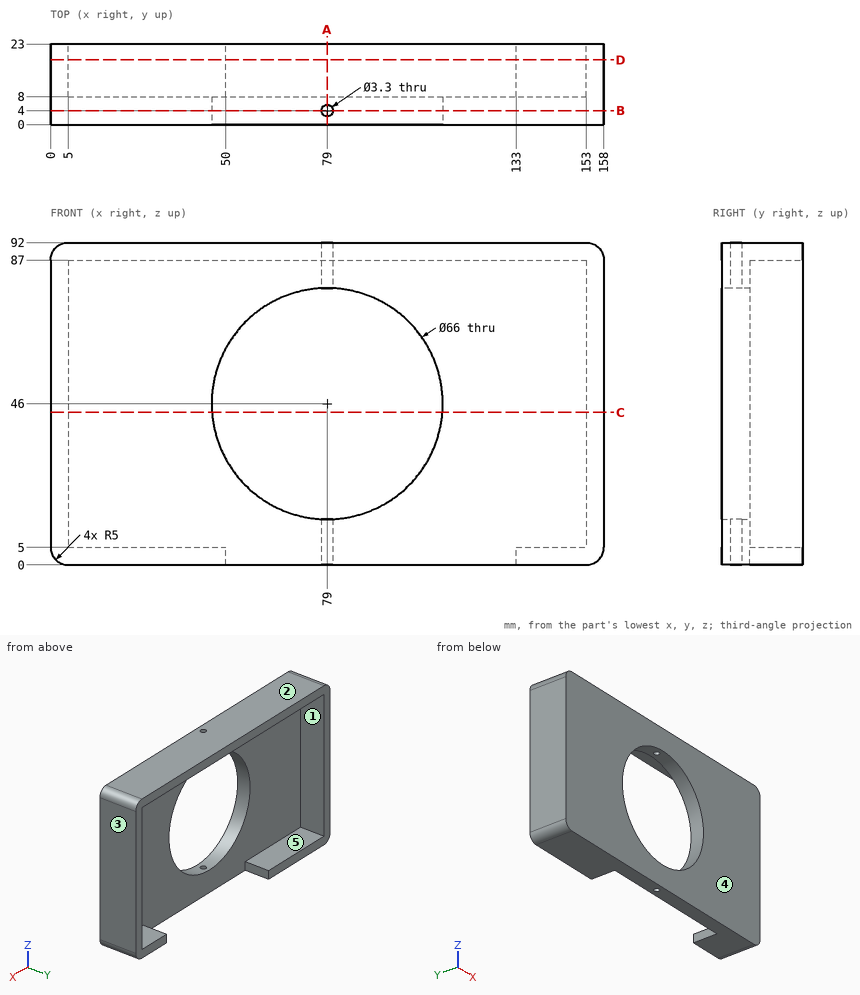
Part print with two shaded views. Sizes in mm from the minimum x, y, z corner. A direction names the side the tool comes from. Round coordinates to 2 decimals unless told otherwise and drop trailing zeros. Order: outer loops, then holes, each group sorted by start corner. A loop starts at its lowest first (then second) coordinate and runs counter-clockwise, first axis right, second up.
(1) Pull direction X, two halves, no side cores. Call the marked faces 1, 2 and 3: released by +X, released by -X, zero draft, split by the parting line, or undercut.
(2) Band-saw the part on A-A (x = 79). List the corners of the cut face in (y, z), then the cut area to 3 significant figures.
(3) 3-axis set-ups, long thin cutter, end or side, ignore diameter. For the marked faces 4 and 5: which of +Z, -Z, +X, -X, +Y, -Y reach the whole face in a straight line?
(4) Band-saw the part on B-B (y = 4). List the corners of the cut face in (x, z), then the cut area to 3 significant figures.
(5) Drill centre lines: line 1 (Y direction, x = 79, z = 10); line 2 (Z direction, x = 29, y = 17); line 3 (X direction, y = 11.5, z = 73.5). Where is each one in solid material? Low to high.
(6) Band-saw the part on C-C (z = 43.5). List the corners of the cut face in (x, y).
(7) Pin check, flat tips, straight feed: pin 1 (5.5 mm diameter, centred on y = 12.5, z = 1.5, fed in from +X); pin 2 (5.5 mm diameter, centred on y = 16, z = 1.5, fed in from -X); pin 3 (6 mm diameter, centred on x = 16, z = 20.5, fed in from +Y). Stop position of each tip, or through.
(8) Band-saw the part on D-D (y = 18.5). List the corners of the cut face in (x, z).
Verdict:
1. face 1: undercut
1. face 2: zero draft
1. face 3: released by +X
2. outline: (0, 0) - (2.35, 0) - (2.35, 13) - (0, 13) - close; (0, 79) - (2.35, 79) - (2.35, 92) - (0, 92) - close; (5.65, 0) - (8, 0) - (8, 13) - (5.65, 13) - close; (5.65, 79) - (8, 79) - (8, 87) - (23, 87) - (23, 92) - (5.65, 92) - close
2. area: 197 mm2
3. face 4: +Z, -Z, +X, -X, -Y
3. face 5: +Y
4. outline: (0, 5) arc R5 ccw to (5, 0) - (77.35, 0) - (77.35, 13.04) arc R33 cw to (77.35, 78.96) - (77.35, 92) - (5, 92) arc R5 ccw to (0, 87) - close; (80.65, 0) - (153, 0) arc R5 ccw to (158, 5) - (158, 87) arc R5 ccw to (153, 92) - (80.65, 92) - (80.65, 78.96) arc R33 cw to (80.65, 13.04) - close
4. area: 11,000 mm2
5. line 1: y = 0 to 2.35, 5.65 to 8
5. line 2: z = 0 to 5, 87 to 92
5. line 3: x = 0 to 5, 153 to 158
6. outline: (0, 0) - (46.09, 0) - (46.09, 8) - (5, 8) - (5, 23) - (0, 23) - close; (111.91, 0) - (158, 0) - (158, 23) - (153, 23) - (153, 8) - (111.91, 8) - close
7. pin 1: stops at x = 157.94
7. pin 2: stops at x = 0.06
7. pin 3: stops at y = 8
8. outline: (0, 5) arc R5 ccw to (5, 0) - (50, 0) - (50, 5) - (5, 5) - (5, 87) - (153, 87) - (153, 5) - (133, 5) - (133, 0) - (153, 0) arc R5 ccw to (158, 5) - (158, 87) arc R5 ccw to (153, 92) - (5, 92) arc R5 ccw to (0, 87) - close
